Design review of the part built by this model. Coordinates are the model's own, in mm. A direction names the side the tool comes from. Coordinates: 2 decimals unless noted, no trailing zeros. Loops run counter-clockwise (first coordinate to the right, second up) from the corner with the lowest first, then second, coordinate; pieces in that order, holes last. Notation, with made-up numbers: M -6.75,65.5 L 49.25,65.5 A25 cw 49.25,94.5 Z; hole C 86.25,-25 d10. An arc over 180 degrees is marked long. Put each result on its own line as item: value. Start each with the question number.
(1) The part is to be moulded in two halves that separate along Z. For faces 5 (the flat face through (0, 0, 7)), 6 (the cylindrical face through (24.542, 13.332, 3.773)), 7 (the flat face through (21.5, -11, 3)), 8 (the flat face through (31.5, 0, 3)), say which applies: +Z half, -Z half, draft (parallel to the pull), parting line (faces both ways), or undercut.
(2) Take a section at A-A, the plane x = -14. Give the boundary of the cut face in (y, z), then the cut area to 3 significant figures.
(3) Take a section at C-C, the plane y = 11.25. Give the boundary of the cut face in (x, z).
(4) For faces 1 (the flat face through (29, 7.5, 3)), 2 (the flat face through (29, 0, 5.5)), 3 (the cylindrical face through (-24.542, 13.332, 3.773)), 4 (the flat face through (-12, 6, 1)), list the 3-axis set-ups (+Z, -Z, +X, -X, +Y, -Y) from which the entire face can be reached by the end or side of a thin tool; tool diameter is ignored.
(5) For probe 1 along Y at (x, z) = (-24.2, 3.5); probe 2 along Y at (x, z) = (-14, 2.75); probe 3 along X at (y, z) = (-4, 4), list the stretches that pass through material, from the lowest coordinate up. Write a range as [from, to].
(6) Clearance check with flat-ended pins moving along their axes: pin 1 (12.5 mm diameter, centred on x = -14, y = 0, fed in from +Z); pin 2 (1.2 mm diameter, centred on x = 30, y = 1.5, fed in from -Z); pin 3 (4 mm diameter, centred on y = -11.25, z = 3.5, fed in from -X). State where each tip first meets the part, or that it passes through.
```python
from build123d import *

# Parameters (mm, degrees)
SKETCH_1_W          = 55
SKETCH_1_H          = 30
SKETCH_1_R          = 7.05
EXTRUDE_1_DEPTH     = 7
SKETCH_2_R          = 7.05
SKETCH_2_R_2        = 6.05
EXTRUDE_2_DEPTH     = 1
EXTRUDE_START       = 1.5
SKETCH_3_W          = 4
SKETCH_3_H          = 15
EXTRUDE_3_DEPTH     = 4
SKETCH_4_R          = 2.1
CUT_EXTRUDE_1_DEPTH = 6


with BuildPart() as part:
    # Эскиз1 → Бобышка-Вытянуть1 (new body)
    with BuildSketch(Plane.XY):
        Rectangle(SKETCH_1_W, SKETCH_1_H)
        with Locations((-14, 0)):
            Circle(SKETCH_1_R, mode=Mode.SUBTRACT)
    extrude(amount=EXTRUDE_1_DEPTH)

    # Эскиз2 → Бобышка-Вытянуть2 (add)
    with BuildSketch(Plane.XY):
        with Locations((-14, 0)):
            Circle(SKETCH_2_R)
        with Locations((-14, 0)):
            Circle(SKETCH_2_R_2, mode=Mode.SUBTRACT)
    extrude(amount=EXTRUDE_2_DEPTH)

    # Эскиз3 → Бобышка-Вытянуть3 (add)
    with BuildSketch(Plane.XY.offset(EXTRUDE_START)):
        with Locations((29.5, 0)):
            Rectangle(SKETCH_3_W, SKETCH_3_H)
        with Locations((-29.5, 0)):
            Rectangle(SKETCH_3_W, SKETCH_3_H)
    extrude(amount=EXTRUDE_3_DEPTH)

    # Эскиз4 → Вырез-Вытянуть1 (cut)
    with BuildSketch(Plane(origin=(27.5, 0, 0), x_dir=(0, 0, -1), z_dir=(1, 0, 0))):
        with Locations((-3.5, 11.25)):
            Circle(SKETCH_4_R)
        with Locations(Location((-3.5, -11.25, 0), (0, 0, 180))):
            Circle(SKETCH_4_R)
    cut_extrude_1 = extrude(amount=-CUT_EXTRUDE_1_DEPTH, mode=Mode.SUBTRACT)

    # Зеркальное отражение1: Вырез-Вытянуть1 across plane
    add(cut_extrude_1.mirror(Plane(origin=(0, 0, 0), x_dir=(0, 0, 1), z_dir=(1, 0, 0))), mode=Mode.SUBTRACT)


solid = part.part
```
Computed values:
1. face 5: +Z half
1. face 6: undercut
1. face 7: undercut
1. face 8: draft
2. outline: M -15,0 L -6.05,0 L -6.05,1 L -7.05,1 L -7.05,7 L -15,7 Z; M 6.05,0 L 15,0 L 15,7 L 7.05,7 L 7.05,1 L 6.05,1 Z
2. area: 113 mm^2
3. outline: M -27.5,0 L 27.5,0 L 27.5,1.4 L 21.5,1.4 L 21.5,5.6 L 27.5,5.6 L 27.5,7 L -27.5,7 L -27.5,5.6 L -21.5,5.6 L -21.5,1.4 L -27.5,1.4 Z
4. face 1: +Z, -Z, +X, +Y
4. face 2: +Z, +X, +Y, -Y
4. face 3: -X
4. face 4: +Z
5. probe 1: y = [-15, -13.35], [-9.15, 9.15], [13.35, 15]
5. probe 2: y = [-15, -7.05], [7.05, 15]
5. probe 3: x = [-31.5, -19.81], [-8.19, 31.5]
6. pin 1: stops at z = 1
6. pin 2: stops at z = 1.5
6. pin 3: stops at x = -21.5
